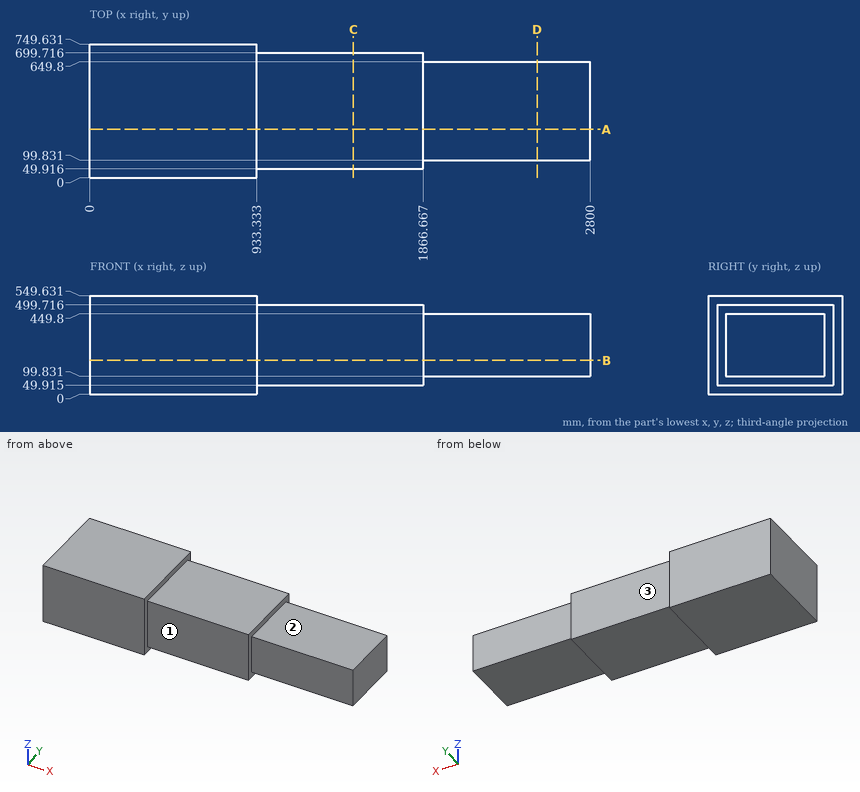
Study the drawing (mm; zero at the part's minimum x, y, z) and answer. A direction names the side the tool comes from. Give positions to 0.01 mm unless a question says otherwise; leave off trailing zeros. Write each loop counter-clockwise with the first axis right and the second up, starting at its lowest first coordinate (ties: lowest second). Pieces come first, ordered by that corner, then holes. Notation, with made-up numbers: (36, 69.25) -> (59, 69.25) arc R22 ccw to (59, 83.25) -> close; hole circle Ø3 at (-17, -20.5). An arc over 180 degrees is marked (long way). Answer as a JSON object with one key per item and string values. Group by question number.
1) Find section C-C (x = 1474.5). Write down the section's boundary in (y, z) (1 decimal), and give its area (3 significant figures).
2) A tool of negligible diameter and unlimited length cuts with its end or side. For the marked faces 1, 2 and 3, from which of +Z, -Z, +X, -X, +Y, -Y can it reach the whole face along a straight path? Write none if from no direction.
3) Find section B-B (z = 188.5). Write down the section's boundary in (x, y) (1 decimal).
4) Find section D-D (x = 2503.5). Write down the section's boundary in (y, z), and give its area (3 significant figures).
5) Find section A-A (y = 271). Write down the section's boundary in (x, z) (1 decimal), and give its area (3 significant figures).
6) Each of these flat-tipped pins is pushed along its axis until it touches: P1, Ø8, axis at x = 2230.5, z = 375, coming from the +Y side; P2, Ø10, axis at x = 1242, y = 350.5, coming from the -Z side (1 decimal). Where does it stop, or does it pass through?
7) Consider L1, parallel to Z at x = 1611, y = 648 (1 decimal); L2, parallel to Z at x = 2307, y = 602; L3, parallel to Y at x = 1266, z = 407 (1 decimal). Determine where each line is inside the solid, lowest interval first. Write a range as from..to.
Values follow:
{
 "1": {"outline": "(49.9, 49.9) -> (699.7, 49.9) -> (699.7, 499.7) -> (49.9, 499.7) -> close", "area": "292,000 mm2"},
 "2": {"face 1": "+Z, -Z, +X, -Y", "face 2": "+Z, +X, +Y, -Y", "face 3": "+Z, -Z, +X, +Y"},
 "3": {"outline": "(0, 0) -> (933.3, 0) -> (933.3, 49.9) -> (1866.7, 49.9) -> (1866.7, 99.8) -> (2800, 99.8) -> (2800, 649.8) -> (1866.7, 649.8) -> (1866.7, 699.7) -> (933.3, 699.7) -> (933.3, 749.6) -> (0, 749.6) -> close"},
 "4": {"outline": "(99.83, 99.83) -> (649.8, 99.83) -> (649.8, 449.8) -> (99.83, 449.8) -> close", "area": "192,000 mm2"},
 "5": {"outline": "(0, 0) -> (933.3, 0) -> (933.3, 49.9) -> (1866.7, 49.9) -> (1866.7, 99.8) -> (2800, 99.8) -> (2800, 449.8) -> (1866.7, 449.8) -> (1866.7, 499.7) -> (933.3, 499.7) -> (933.3, 549.6) -> (0, 549.6) -> close", "area": "1,260,000 mm2"},
 "6": {"P1": "stops at y = 649.8", "P2": "stops at z = 49.9"},
 "7": {"L1": "z = 49.9..499.7", "L2": "z = 99.83..449.8", "L3": "y = 49.9..699.7"}
}
